Input: dimensioned drawing with shaded views. Units: mm. Origin: part minimum x, y, z. Coordinates: 2 decimals unless noted, no trailing zeros. Loops run counter-clockwise (first coordinate to the right, second up) from the corner with the lowest first, then second, coordinate; pieces in that order, holes last.
Item 1: Section B-B on z = 7. Return loops of the section in (x, y).
Item 2: Section A-A on y = 6.35. Give the number of separate pieces and of enclosed holes in the cut face, and give its area (3 significant figures).
Item 3: Ray query, line 1 along X through (y, z) = (6.35, 0.5); line 2 along Z through (x, y) = (223.5, 4). Return the intervals inside material, ascending.
Item 4: Section C-C on x = 305. Return loops of the section in (y, z), and give its area (3 significant figures).
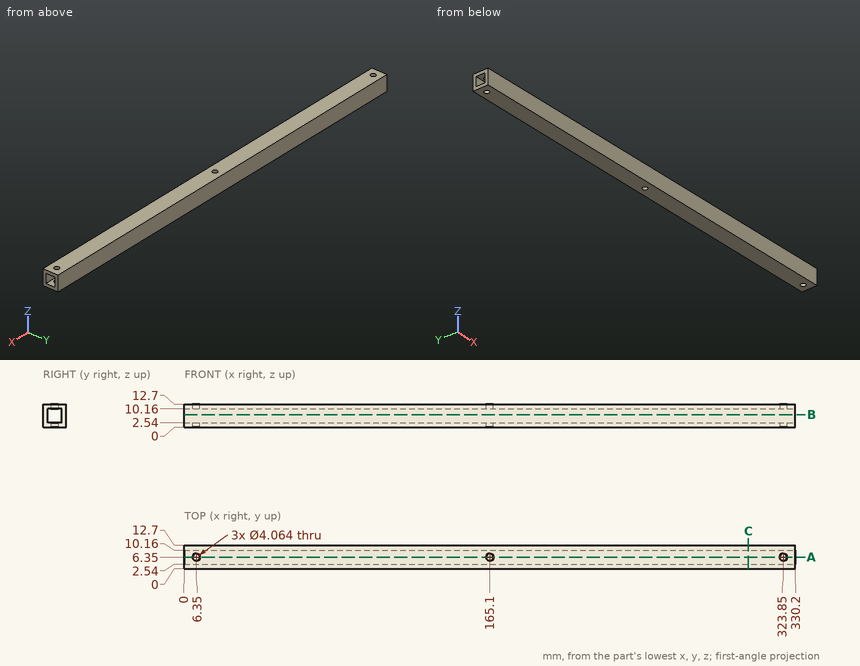
Results found:
1. outline: (0, 0) - (330.2, 0) - (330.2, 2.54) - (0, 2.54) - close; (0, 10.16) - (330.2, 10.16) - (330.2, 12.7) - (0, 12.7) - close
2. separate pieces: 8
2. enclosed holes: 0
2. area: 1,620 mm2
3. line 1: x = 0 to 4.32, 8.38 to 163.07, 167.13 to 321.82, 325.88 to 330.2
3. line 2: z = 0 to 2.54, 10.16 to 12.7
4. outline: (0, 0) - (12.7, 0) - (12.7, 12.7) - (0, 12.7) - close; hole (2.54, 2.54) - (10.16, 2.54) - (10.16, 10.16) - (2.54, 10.16) - close
4. area: 103 mm2
